from build123d import *

# Parameters (mm, degrees)
F0_R     = 20
F0_R_2   = 19
F1_DEPTH = 1
F2_R     = 20
F3_DEPTH = 1.5
F4_R     = 0.5
F5_DEPTH = 2.501
F6_R     = 0.9
F7_DEPTH = 1


with BuildPart() as f1:
    # F0 (on Top) → F1 (new body)
    with BuildSketch(Plane.XY):
        Circle(F0_R)
        Circle(F0_R_2, mode=Mode.SUBTRACT)
    extrude(amount=F1_DEPTH)

    # F2 (on face) → F3 (join)
    with BuildSketch(Plane.XY.offset(1)):
        Circle(F2_R)
    extrude(amount=F3_DEPTH)

    # F4 (on face) → F5 (cut, through all)
    with BuildSketch(Plane.XY.offset(2.5)):
        with Locations((0, 18)):
            Circle(F4_R)
        with Locations((15.5884572681, 9)):
            Circle(F4_R)
        with Locations((15.5884572681, -9)):
            Circle(F4_R)
        with Locations((0, -18)):
            Circle(F4_R)
        with Locations((-15.5884572681, -9)):
            Circle(F4_R)
        with Locations((-15.5884572681, 9)):
            Circle(F4_R)
    extrude(amount=-F5_DEPTH, mode=Mode.SUBTRACT)

    # F6 (on face) → F7 (cut)
    with BuildSketch(Plane.XY.offset(2.5)):
        with Locations((0, 18)):
            Circle(F6_R)
        with Locations((-15.5884572681, 9)):
            Circle(F6_R)
        with Locations((-15.5884572681, -9)):
            Circle(F6_R)
        with Locations((0, -18)):
            Circle(F6_R)
        with Locations((15.5884572681, -9)):
            Circle(F6_R)
        with Locations((15.5884572681, 9)):
            Circle(F6_R)
    extrude(amount=-F7_DEPTH, mode=Mode.SUBTRACT)

    # F8 (on Right) → F9 (revolve, cut)
    with BuildSketch(Plane.YZ):
        with BuildLine():
            Line((20, 1.5), (20, 2.5))
            Line((20, 2.5), (19, 2.5))
            ThreePointArc((19, 2.5), (19.7071067812, 2.2071067812), (20, 1.5))
        make_face()
    revolve(axis=Axis((0, 0, 3.847687738), (0, 0, 1)), mode=Mode.SUBTRACT)


solid = f1.part
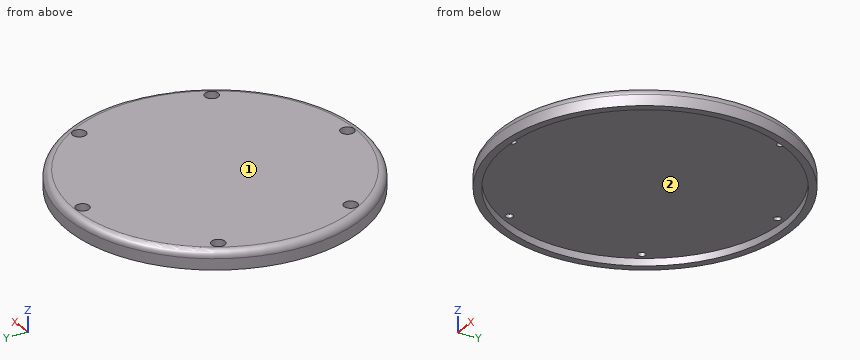
Part model, mm, in its own coordinate system. Face numbers are marked on the shaded views. Coordinates: 2 decimals unless noted, no trailing zeros. Order: outer loops, then holes, each group sorted by start corner. A loop starts at its lowest first (then second) coordinate and runs counter-clockwise, first axis right, second up.
(1) Slice it at D-D, the plane y = 9. State how many separate pieces and enclosed holes the cut face has, and give its area (3 significant figures).
Check sheet entries:
separate pieces: 3
enclosed holes: 0
area: 50.8 mm2
(2) Slice it at C-C, the plane y = 0. Write the cut outline in (x, z), and give its area (3 significant figures).
Check sheet entries:
outline: (-20, 0) - (-19, 0) - (-19, 1) - (19, 1) - (19, 0) - (20, 0) - (20, 1.5) arc R1 ccw to (19, 2.5) - (-19, 2.5) arc R1 ccw to (-20, 1.5) - close
area: 61.6 mm2
(3) Slice it at A-A, the plane z = 2.1. Write the cut outline in (x, y).
Check sheet entries:
outline: circle Ø39.6 at (0, 0); hole circle Ø1.8 at (-15.59, -9); hole circle Ø1.8 at (-15.59, 9); hole circle Ø1.8 at (0, -18); hole circle Ø1.8 at (0, 18); hole circle Ø1.8 at (15.59, -9); hole circle Ø1.8 at (15.59, 9)
(4) Probe L1, parallel to Y at x = 0, z = 1.2; L2, parallel to Y at x = 0, z = 2.05; L3, parallel to Z at x = -13, y = 10.5. List the from-to ranges inside material, lowest first.
Check sheet entries:
L1: y = -20 to -18.5, -17.5 to 17.5, 18.5 to 20
L2: y = -19.84 to -18.9, -17.1 to 17.1, 18.9 to 19.84
L3: z = 1 to 2.5
(5) Slice it at B-B, the plane x = 0. Write the cut outline in (y, z).
Check sheet entries:
outline: (-20, 0) - (-19, 0) - (-19, 1) - (-18.5, 1) - (-18.5, 1.5) - (-18.9, 1.5) - (-18.9, 2.5) - (-19, 2.5) arc R1 ccw to (-20, 1.5) - close; (-17.5, 1) - (17.5, 1) - (17.5, 1.5) - (17.1, 1.5) - (17.1, 2.5) - (-17.1, 2.5) - (-17.1, 1.5) - (-17.5, 1.5) - close; (18.5, 1) - (19, 1) - (19, 0) - (20, 0) - (20, 1.5) arc R1 ccw to (19, 2.5) - (18.9, 2.5) - (18.9, 1.5) - (18.5, 1.5) - close
(6) Pull direction X, two halves, no side cores. Call the marked faces 1 and 2: pulls with the +X half, pulls with the -X half, needs draft (parallel to the pull), parting line crosses it, or undercut.
Check sheet entries:
face 1: needs draft
face 2: undercut
(7) Pin check, flat tips, straight feed: pin 1 Ø1.6 at (x, y) = (15.59, -9) entering from -Z; pin 2 Ø1.6 at (x, y) = (0, -18) entering from +Z. Stop position of each tip, or through.
Check sheet entries:
pin 1: stops at z = 1
pin 2: stops at z = 1.5
